Study the drawing (mm; zero at the part's minimum x, y, z) and answer. A direction names the side the tool comes from. Round coordinates to 2 decimals unless told otherwise and drop trailing zeros. Order: outer loops, then holes, each group sorted by start corner. A loop starts at its lowest first (then second) coordinate and runs counter-clockwise, first axis right, second up. Notation, with made-up numbers: (-24, -27) - (0, -27) arc R31 ccw to (0, 0) - close; hole circle Ø7 at (-30.5, 22.5). An arc over 180 degrees is marked (long way). Use one line per item in the form item = value. Start each with the question number.
Q1. The part is cut by section D-D on x = 4.5. Determine the outline of the cut face in (y, z), plus the area to 3 significant figures.
Q2. The part is cut by section C-C on z = 7.75. Determine the outline of the cut face in (x, y).
Q3. For a pull along Y with two mould halves and no side action, classify the marked faces 4, 5 and 6 as +Y half, -Y half, draft (parallel to the pull), parting line (faces both ways), or undercut.
Q4. Given P1, Ø1, axis at x = 21.5, z = 21, coming from the -Y side; P2, Ø10, axis at x = 29, z = 12.5, coming from the -Y side; P3, Ø1, axis at x = 22.5, y = 3, coming from the -Z side (1 decimal), each flat-ended and moving along its own axis, determine where each tip first touches the part or whether it passes through.
Q5. Which of the six approach directions +Z, -Z, +X, -X, +Y, -Y give full straight-line access (tool end or side, diameter ignored) to the marked faces 1, 2 and 3?
Q6. The part is cut by section B-B on y = 15.25. Determine the outline of the cut face in (x, z), plus the area to 3 significant figures.
Q7. Find the intervals of material crossed by line 1 (Z direction, x = 14.5, y = 11) (1 decimal); line 2 (Y direction, x = 28.5, z = 9.5) (1 decimal); line 3 (Y direction, x = 23, z = 17.5) (1 decimal), in increasing order. Write a range as [from, to].
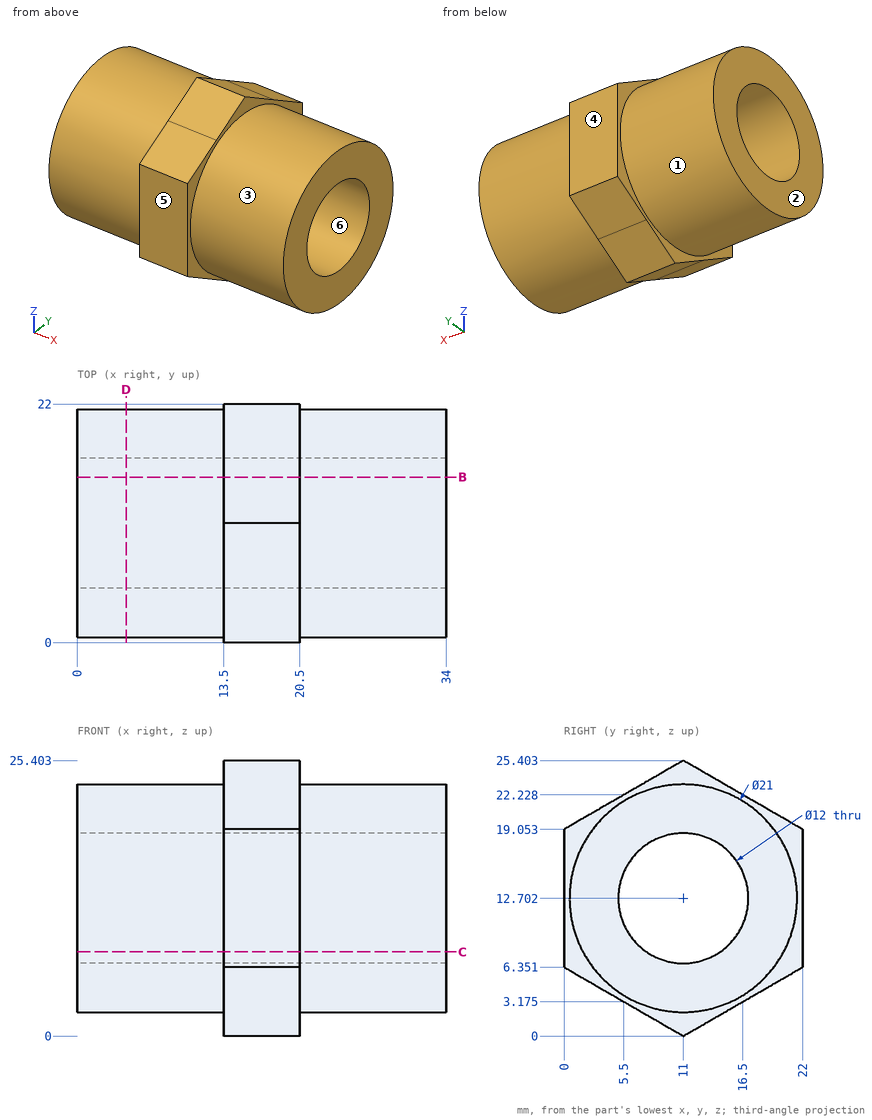
Found:
q1.outline = circle Ø21 at (11, 12.7); hole circle Ø12 at (11, 12.7)
q1.area = 233 mm²
q2.outline = (0, 1.74) - (13.5, 1.74) - (13.5, 0) - (20.5, 0) - (20.5, 1.74) - (34, 1.74) - (34, 7.61) - (0, 7.61) - close; (0, 14.39) - (34, 14.39) - (34, 20.26) - (20.5, 20.26) - (20.5, 22) - (13.5, 22) - (13.5, 20.26) - (0, 20.26) - close
q3.face_4 = +Y half
q3.face_5 = -Y half
q3.face_6 = undercut
q4.P1 = 3.97
q4.P2 = 0.5
q4.P3 = 5.4
q5.face_1 = -X
q5.face_2 = +Z, -Z, -X, +Y, -Y
q5.face_3 = +X
q6.outline = (0, 3.1) - (13.5, 3.1) - (13.5, 2.45) - (20.5, 2.45) - (20.5, 3.1) - (34, 3.1) - (34, 8.47) - (0, 8.47) - close; (0, 16.94) - (34, 16.94) - (34, 22.3) - (20.5, 22.3) - (20.5, 22.95) - (13.5, 22.95) - (13.5, 22.3) - (0, 22.3) - close
q6.area = 374 mm²
q7.line_1 = [0, 6.7], [18.7, 25.4]
q7.line_2 = [1, 5.9], [16.1, 21]
q7.line_3 = [1.7, 7.4], [14.6, 20.3]
